Check sheet for the modelled part. Datum: model origin and axes. Units: mm. A direction names the side the tool comes from. Give positions to 0.01 mm unless a question says otherwise; leave off trailing zeros. Order: outer loops, then holes, each group sorted by start corner. A loop starts at its lowest first (then second) coordinate and runs counter-clockwise, first axis right, second up. Notation, with made-up numbers: M 32.25,89 L 50.25,89 A19 cw 50.25,103 Z; hole C 55.25,54.5 d9. An arc over 180 degrees is marked long. Return JSON: item names as keys, results as strings. Group by question number.
from build123d import *

# Parameters (mm, degrees)
SKICA1_R                = 7
P_IDAT_VYSUNUT_M1_DEPTH = 3
SKICA2_R                = 5
P_IDAT_VYSUNUT_M2_DEPTH = 25
ZAOBLIT1_R              = 1


with BuildPart() as part:
    # Skica1 → Přidat vysunutím1 (new body)
    with BuildSketch(Plane.XY):
        Circle(SKICA1_R)
    extrude(amount=P_IDAT_VYSUNUT_M1_DEPTH)

    # Skica2 → Přidat vysunutím2 (add)
    with BuildSketch(Plane(origin=(0, 0, 0), x_dir=(-1, 0, 0), z_dir=(0, 0, -1))):
        Circle(SKICA2_R)
    extrude(amount=P_IDAT_VYSUNUT_M2_DEPTH)

    # Zaoblit1
    zaoblit1_edges = [part.edges().sort_by_distance(p)[0] for p in [
        (-7, 0, 3),
        (5, 0, -25),
    ]]
    fillet(zaoblit1_edges, radius=ZAOBLIT1_R)


solid = part.part
1) Tool access check on faces 1 (the face through (-2, 5, 0)), 2 (the face through (6.466, -2.681, 0.986)). Record the directions out of +Z, -Z, +X, -X, +Y, -Y that give a thin tool (end or side, any length) a straight path to the whole face; none if there is none.
2) Sectioned sample at C-C on z = -16. Record the boundary of the cut face in (x, y), then the cut area to 3 significant figures.
3) Sectioned sample at A-A on y = 0. Record the boundary of the cut face in (x, z), then the cut area to 3 significant figures.
4) Material ranges on line 1 along Y through (x, z) = (3, -5); line 2 along Z through (x, y) = (5.25, 0); line 3 along Z through (x, y) = (-4, -1), recorded low to high.
5) Depth check by flat-ended pin: P1, Ø2, axis at y = -5.5, z = -12, coming from the +X side; P2, Ø1.5, axis at y = -1, z = -9, coming from the +X side; P3, Ø3, axis at x = 2.5, z = -9, coming from the +Y side. Enter the tip coordinate at first touch or a pass-through.
Reply:
{
 "1": {"face 1": "-Z", "face 2": "+Z, -Z"},
 "2": {"outline": "C 0,0 d10", "area": "78.5 mm^2"},
 "3": {"outline": "M -7,0 L -5,0 L -5,-24 A1 ccw -4,-25 L 4,-25 A1 ccw 5,-24 L 5,0 L 7,0 L 7,2 A1 ccw 6,3 L -6,3 A1 ccw -7,2 Z", "area": "291 mm^2"},
 "4": {"line 1": "-4 to 4", "line 2": "0 to 3", "line 3": "-24.99 to 3"},
 "5": {"P1": "x = 2.18", "P2": "x = 4.99", "P3": "y = 4.9"}
}
